Could you check a few things on this model? Use its own coordinates, in mm. A direction names the side the tool comes from. Coordinates: 2 decimals unless noted, no trailing zeros. Order: outer loops, then holes, each group sorted by start corner. A loop starts at its lowest first (then second) coordinate and runs counter-clockwise, first axis right, second up. Notation, with made-up numbers: M 29,-8.75 L 40,-8.75 A19 ccw 40,28.25 Z; hole C 65.25,-27 d1. An arc over 180 degrees is marked long. Put each result on its own line as item: value. Start each with the question number.
```python
from build123d import *

# Parameters (mm, degrees)
F1_DEPTH = 7.29556
F2_R     = 3.352676
F2_R_2   = 3.043736
F3_DEPTH = 25.4
F4_R     = 2.721631
F4_R_2   = 2.684235
F5_DEPTH = 25.4
F6_R     = 5.08
F7_R     = 5.08


with BuildPart() as f1:
    # F0 (on Top) → F1 (new body)
    with BuildSketch(Plane.XY):
        Polygon((-57.594109, -42.704724), (-57.594109, -54.158099), (5.890307, -54.158099), (5.890307, -42.704724), (-11.126135, 0), (-11.126135, 10.962515), (-37.959754, 10.962515), (-37.959754, 0), align=None)
    extrude(amount=F1_DEPTH)

    # F2 (on Top) → F3 (cut)
    with BuildSketch(Plane.XY):
        with Locations((-31.249143, 5.297316)):
            Circle(F2_R)
        with Locations((-18.129976, 5.297316)):
            Circle(F2_R_2)
    extrude(amount=F3_DEPTH, mode=Mode.SUBTRACT)

    # F4 (on Top) → F5 (cut)
    with BuildSketch(Plane.XY):
        with Locations((-51.31226, -47.847249)):
            Circle(F4_R)
        with Locations((0, -47.847249)):
            Circle(F4_R_2)
    extrude(amount=F5_DEPTH, mode=Mode.SUBTRACT)

    # F6
    f6_edges = [f1.edges().sort_by_distance(p)[0] for p in [
        (-57.594109, -54.158099, 3.64778),
        (5.890307, -54.158099, 3.64778),
    ]]
    fillet(f6_edges, radius=F6_R)

    # F7
    f7_edges = [f1.edges().sort_by_distance(p)[0] for p in [
        (-37.959754, 10.962515, 3.64778),
        (-11.126135, 10.962515, 3.64778),
    ]]
    fillet(f7_edges, radius=F7_R)


solid = f1.part
```
Item 1: If we section it at B-B on z = 3: Write out the boundary of the cut face in (x, y).
Item 2: If we section it at C-C on x = -51: Write out the boundary of the cut face in (y, z), then the cut area to 3 significant figures.
Item 3: For pin 1 Ø2 at (y, z) = (-19.5, 2) entering from +X; pin 2 Ø1.8 at (y, z) = (3, 4) entering from +X; pin 3 Ø1 at (y, z) = (-16.5, 6) entering from -X, each with a flat end and sliding along its axis, tell me the tip position at first contact or that it passes through.
Item 4: For faces 5 (the flat face through (-37.96, 3, 4)), 6 (the flat face through (-57.594, -46, 4)), 7 (the flat face through (-11.126, 3, 4)), which set-ups out of +Z, -Z, +X, -X, +Y, -Y let a thin tool reach every point of the face, with its end or its side?
Item 5: If we section it at D-D on y = -15: Write out the boundary of the cut face in (x, z).
Item 6: If we section it at A-A on x = 0: Write out the boundary of the cut face in (y, z), then the cut area to 3 significant figures.
Item 7: If we mould it in two halves opening along X, with no side actions, what happens to faces 1 (the cylindrical face through (-51.67, -45.15, 3.6)), 2 (the flat face through (5.89, -46, 4)), 3 (the cylindrical face through (-36.511, 9.435, 3.699)), 4 (the cylindrical face through (-20.55, 3.45, 3.6))? For each: released by +X, released by -X, zero draft, split by the parting line, or undercut.
Item 8: I need wall thicknesses on probe 1 along X at (y, z) = (-47.5, 7.25); probe 2 along X at (y, z) = (3, 2.75); probe 3 along X at (y, z) = (0, 5.5). Which ranges of each line are inside material? Lowest first, please.
Geometry check:
1. outline: M -57.59,-49.08 A5.08 ccw -52.51,-54.16 L 0.81,-54.16 A5.08 ccw 5.89,-49.08 L 5.89,-42.7 L -11.13,0 L -11.13,5.88 A5.08 ccw -16.21,10.96 L -32.88,10.96 A5.08 ccw -37.96,5.88 L -37.96,0 L -57.59,-42.7 Z; hole C -51.31,-47.85 d5.44; hole C -31.25,5.3 d6.71; hole C -18.13,5.3 d6.09; hole C 0,-47.85 d5.37
2. outline: M -54.16,0 L -50.55,0 L -50.55,7.3 L -54.16,7.3 Z; M -45.14,0 L -28.36,0 L -28.36,7.3 L -45.14,7.3 Z
2. area: 149 mm²
3. pin 1: stops at x = -2.96
3. pin 2: stops at x = -11.13
3. pin 3: stops at x = -45.78
4. face 5: +Z, -Z, -X, +Y
4. face 6: +Z, -Z, -X, +Y, -Y
4. face 7: +Z, -Z, +X, +Y
5. outline: M -44.86,0 L -5.15,0 L -5.15,7.3 L -44.86,7.3 Z
6. outline: M -54.16,0 L -50.53,0 L -50.53,7.3 L -54.16,7.3 Z; M -45.16,0 L -27.92,0 L -27.92,7.3 L -45.16,7.3 Z
6. area: 152 mm²
7. face 1: undercut
7. face 2: released by +X
7. face 3: released by -X
7. face 4: undercut
8. probe 1: x = -57.59 to -54.01, -48.61 to -2.66, 2.66 to 5.89
8. probe 2: x = -37.96 to -33.69, -28.81 to -20.13, -16.13 to -11.13
8. probe 3: x = -37.96 to -11.13
